Part print with two shaded views. Sizes in mm from the minimum x, y, z corner. A direction names the side the tool comes from. Round coordinates to 2 decimals unless told otherwise and drop trailing zeros. Loops run counter-clockwise (first coordinate to the right, second up) from the corner with the lowest first, then second, coordinate; pieces in that order, holes last. Notation, with made-up numbers: (-18.75, 71.5) -> (-7.75, 71.5) arc R31 cw to (-7.75, 103.5) -> close; hole circle Ø2 at (36.25, 58.25). An arc over 180 degrees is marked (long way). Use a Markdown table: item, result. Add a question column.
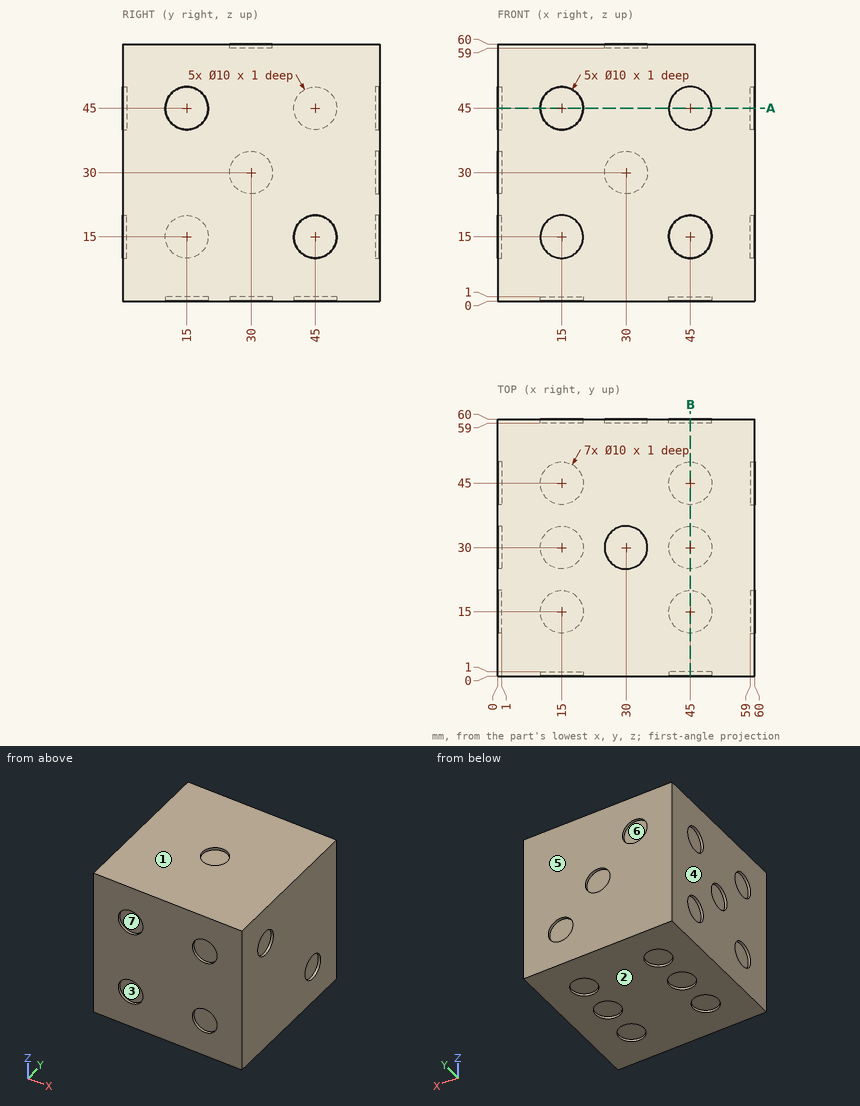
1) Wall check: probe 1 along X at (y, z) = (0.55, 15); probe 2 along Z at (x, y) = (15, 48). Give the ranges that are in metal, low to high. Write a range as from..to.
2) Pin check, flat tips, straight feed: pin 1 Ø8 at (x, y) = (45, 45) entering from -Z; pin 2 Ø9 at (x, y) = (30, 30) entering from +Z; pin 3 Ø3 at (x, z) = (45.5, 43) entering from -Y. Stop position of each tip, or through.
3) Tool access for the marked faces 5, 6 and 7: list every direction of +Z, -Z, +X, -X, +Y, -Y with a clear straight run to the whole face (end or side of a thin tool).
4) Pull direction Z, two halves, no side cores. Call the marked faces 1, 2, 3 and 4: +Z half, -Z half, draft (parallel to the pull), parting line (faces both ways), or undercut.
5) Cut at A-A on z = 45. Write the cut outline in (x, y).
6) Cut at B-B on x = 45. Write the cut outline in (y, z).
Established:
| question | item | result |
|---|---|---|
| 1 | probe 1 | x = 0..10, 20..40, 50..60 |
| 1 | probe 2 | z = 1..60 |
| 2 | pin 1 | stops at z = 1 |
| 2 | pin 2 | stops at z = 59 |
| 2 | pin 3 | stops at y = 1 |
| 3 | face 5 | +Z, -Z, +X, -X, +Y |
| 3 | face 6 | +Y |
| 3 | face 7 | -Y |
| 4 | face 1 | +Z half |
| 4 | face 2 | -Z half |
| 4 | face 3 | undercut |
| 4 | face 4 | draft |
| 5 | outline | (0, 0) -> (10, 0) -> (10, 1) -> (20, 1) -> (20, 0) -> (40, 0) -> (40, 1) -> (50, 1) -> (50, 0) -> (60, 0) -> (60, 10) -> (59, 10) -> (59, 20) -> (60, 20) -> (60, 60) -> (20, 60) -> (20, 59) -> (10, 59) -> (10, 60) -> (0, 60) -> (0, 50) -> (1, 50) -> (1, 40) -> (0, 40) -> (0, 20) -> (1, 20) -> (1, 10) -> (0, 10) -> close |
| 6 | outline | (0, 0) -> (10, 0) -> (10, 1) -> (20, 1) -> (20, 0) -> (25, 0) -> (25, 1) -> (35, 1) -> (35, 0) -> (40, 0) -> (40, 1) -> (50, 1) -> (50, 0) -> (60, 0) -> (60, 10) -> (59, 10) -> (59, 20) -> (60, 20) -> (60, 60) -> (0, 60) -> (0, 50) -> (1, 50) -> (1, 40) -> (0, 40) -> (0, 20) -> (1, 20) -> (1, 10) -> (0, 10) -> close |
